```python
from build123d import *

# Parameters (mm, degrees)
SKETCH1_W                       = 88.9
SKETCH1_H                       = 60.325
BOSS_EXTRUDE1_DEPTH             = 36.5252
CUT_EXTRUDE1_DEPTH              = 30.1752
CUT_EXTRUDE5_DEPTH              = 4.7752
SKETCH3_R                       = 6.0452
CUT_EXTRUDE2_DEPTH              = 65.958980451
CUT_EXTRUDE3_DEPTH              = 3.6576
SKETCH8_OUTSIDE_W               = 113.594
SKETCH8_OUTSIDE_H               = 85.018
CUT_EXTRUDE4_DEPTH              = 28.575
F_10_32_TAPPED_HOLE1_AT_2_COUNT = 2
F_10_32_TAPPED_HOLE1_AT_2_PITCH = 47.6504
F_10_32_TAPPED_HOLE1_AT_3_COUNT = 2
F_10_32_TAPPED_HOLE1_AT_3_PITCH = 76.2
F_10_32_TAPPED_HOLE1_AT_4_COUNT = 2
F_10_32_TAPPED_HOLE1_AT_4_PITCH = 89.872134837
F_6_32_TAPPED_HOLE1_D           = 2.7051
F_6_32_TAPPED_HOLE1_DEPTH       = 9.398
F_6_32_TAPPED_HOLE1_CSINK_D     = 3.81
F_6_32_TAPPED_HOLE1_CSINK_ANGLE = 90
F_6_32_TAPPED_HOLE1_TIP         = 0.81269403
FILLET1_R                       = 3.175
F_8_32_TAPPED_HOLE1_AT_2_COUNT  = 2
F_8_32_TAPPED_HOLE1_AT_2_PITCH  = 9.525


with BuildPart() as part:
    # Sketch1 → Boss-Extrude1 (new body)
    with BuildSketch(Plane.XY):
        Rectangle(SKETCH1_W, SKETCH1_H)
    extrude(amount=-BOSS_EXTRUDE1_DEPTH)

    # Sketch2 → Cut-Extrude1 (cut)
    with BuildSketch(Plane.XY):
        with BuildLine():
            Line((8.699713209, 23.8252), (20.6375, 23.8252))
            ThreePointArc((20.6375, 23.8252), (32.202723567, 16.372637836), (30.194632556, 2.761515566))
            ThreePointArc((30.194632556, 2.761515566), (29.156922747, 0), (30.194632556, -2.761515566))
            ThreePointArc((30.194632556, -2.761515566), (32.202723567, -16.372637836), (20.6375, -23.8252))
            Line((20.6375, -23.8252), (8.699713209, -23.8252))
            Line((8.699713209, -23.8252), (-8.699713209, -23.8252))
            Line((-8.699713209, -23.8252), (-20.6375, -23.8252))
            ThreePointArc((-20.6375, -23.8252), (-32.202723567, -16.372637836), (-30.194632556, -2.761515566))
            ThreePointArc((-30.194632556, -2.761515566), (-29.156922747, 0), (-30.194632556, 2.761515566))
            ThreePointArc((-30.194632556, 2.761515566), (-32.202723567, 16.372637836), (-20.6375, 23.8252))
            Line((-20.6375, 23.8252), (-8.699713209, 23.8252))
            Line((-8.699713209, 23.8252), (8.699713209, 23.8252))
        make_face()
    extrude(amount=-CUT_EXTRUDE1_DEPTH, mode=Mode.SUBTRACT)

    # Sketch9 → Cut-Extrude5 (cut)
    with BuildSketch(Plane.XY):
        with BuildLine():
            Line((-20.6375, -25.4254), (20.6375, -25.4254))
            ThreePointArc((20.6375, -25.4254), (28.764361073, -22.891671397), (34.011365871, -16.188344448))
            Line((34.011365871, -16.188344448), (39.288861577, -2.248287943))
            ThreePointArc((39.288861577, -2.248287943), (39.7002, 0), (39.288861577, 2.248287943))
            Line((39.288861577, 2.248287943), (34.011365871, 16.188344448))
            ThreePointArc((34.011365871, 16.188344448), (28.764361073, 22.891671397), (20.6375, 25.4254))
            Line((20.6375, 25.4254), (-20.6375, 25.4254))
            ThreePointArc((-20.6375, 25.4254), (-28.764361073, 22.891671397), (-34.011365871, 16.188344448))
            Line((-34.011365871, 16.188344448), (-39.288861577, 2.248287943))
            ThreePointArc((-39.288861577, 2.248287943), (-39.7002, 0), (-39.288861577, -2.248287943))
            Line((-39.288861577, -2.248287943), (-34.011365871, -16.188344448))
            ThreePointArc((-34.011365871, -16.188344448), (-28.764361073, -22.891671397), (-20.6375, -25.4254))
        make_face()
    extrude(amount=-CUT_EXTRUDE5_DEPTH, mode=Mode.SUBTRACT)

    # Sketch3 → Cut-Extrude2 (cut, through all)
    with BuildSketch(Plane(origin=(0, 0, -36.5252), x_dir=(-1, 0, 0), z_dir=(0, 0, -1))):
        with Locations((-20.6502, 11.1252)):
            Circle(SKETCH3_R)
        with Locations((-20.6502, -11.1252)):
            Circle(SKETCH3_R)
        with Locations((20.6502, 11.1252)):
            Circle(SKETCH3_R)
        with Locations((20.6502, -11.1252)):
            Circle(SKETCH3_R)
    extrude(amount=-CUT_EXTRUDE2_DEPTH, mode=Mode.SUBTRACT)

    # Sketch4 → Cut-Extrude3 (cut)
    with BuildSketch(Plane.XY):
        with BuildLine():
            Line((20.6375, 28.9814), (-20.6375, 28.9814))
            ThreePointArc((-20.6375, 28.9814), (-30.78525015, 25.817614551), (-37.337016354, 17.447385697))
            Line((-37.337016354, 17.447385697), (-42.61451206, 3.507329192))
            ThreePointArc((-42.61451206, 3.507329192), (-43.2562, 0), (-42.61451206, -3.507329192))
            Line((-42.61451206, -3.507329192), (-37.337016354, -17.447385697))
            ThreePointArc((-37.337016354, -17.447385697), (-30.78525015, -25.817614551), (-20.6375, -28.9814))
            Line((-20.6375, -28.9814), (20.6375, -28.9814))
            ThreePointArc((20.6375, -28.9814), (30.78525015, -25.817614551), (37.337016354, -17.447385697))
            Line((37.337016354, -17.447385697), (42.61451206, -3.507329192))
            ThreePointArc((42.61451206, -3.507329192), (43.2562, 0), (42.61451206, 3.507329192))
            Line((42.61451206, 3.507329192), (37.337016354, 17.447385697))
            ThreePointArc((37.337016354, 17.447385697), (30.78525015, 25.817614551), (20.6375, 28.9814))
        make_face()
    extrude(amount=-CUT_EXTRUDE3_DEPTH, mode=Mode.SUBTRACT)

    # Sketch8 outside → Cut-Extrude4 (cut)
    with BuildSketch(Plane(origin=(0, 0, -36.5252), x_dir=(-1, 0, 0), z_dir=(0, 0, -1))):
        Rectangle(SKETCH8_OUTSIDE_W, SKETCH8_OUTSIDE_H)
        with BuildLine():
            Line((20.6375, -28.6512), (-20.6375, -28.6512))
            ThreePointArc((-20.6375, -28.6512), (-33.030253447, -23.517953447), (-38.1635, -11.1252))
            Line((-38.1635, -11.1252), (-38.1635, 11.1252))
            ThreePointArc((-38.1635, 11.1252), (-33.030253447, 23.517953447), (-20.6375, 28.6512))
            Line((-20.6375, 28.6512), (20.6375, 28.6512))
            ThreePointArc((20.6375, 28.6512), (33.030253447, 23.517953447), (38.1635, 11.1252))
            Line((38.1635, 11.1252), (38.1635, -11.1252))
            ThreePointArc((38.1635, -11.1252), (33.030253447, -23.517953447), (20.6375, -28.6512))
        make_face(mode=Mode.SUBTRACT)
    extrude(amount=-CUT_EXTRUDE4_DEPTH, mode=Mode.SUBTRACT)

    # Sketch6 → #10-32 Tapped Hole1 (revolve, cut)
    with BuildSketch(Plane(origin=(38.1, 23.8252, 0), x_dir=(0, -1, 0), z_dir=(1, 0, 0))):
        Polygon((0, 0), (0, 7.9502), (2.667, 7.9502), (2.0193, 7.3025), (2.0193, 0.6477), (2.667, 0), align=None)
    f_10_32_tapped_hole1 = revolve(axis=Axis((38.1, 23.8252, 6.35), (0, 0, -1)), mode=Mode.SUBTRACT)

    # #10-32 Tapped Hole1 at 2: #10-32 Tapped Hole1 ×2
    with Locations(*[(0, -i * F_10_32_TAPPED_HOLE1_AT_2_PITCH, 0) for i in range(1, F_10_32_TAPPED_HOLE1_AT_2_COUNT)]):
        add(f_10_32_tapped_hole1, mode=Mode.SUBTRACT)

    # #10-32 Tapped Hole1 at 3: #10-32 Tapped Hole1 ×2
    with Locations(*[(-i * F_10_32_TAPPED_HOLE1_AT_3_PITCH, 0, 0) for i in range(1, F_10_32_TAPPED_HOLE1_AT_3_COUNT)]):
        add(f_10_32_tapped_hole1, mode=Mode.SUBTRACT)

    # #10-32 Tapped Hole1 at 4: #10-32 Tapped Hole1 ×2
    with Locations(*[Vector(-0.8478712577397053, -0.5302021598398957, 0) * (i * F_10_32_TAPPED_HOLE1_AT_4_PITCH) for i in range(1, F_10_32_TAPPED_HOLE1_AT_4_COUNT)]):
        add(f_10_32_tapped_hole1, mode=Mode.SUBTRACT)

    # #6-32 Tapped Hole1
    with Locations(Plane.XY.offset(-4.7752)):
        with Locations((33.3502, 0), (-33.3502, 0)):
            CounterSinkHole(F_6_32_TAPPED_HOLE1_D / 2, F_6_32_TAPPED_HOLE1_CSINK_D / 2, depth=F_6_32_TAPPED_HOLE1_DEPTH, counter_sink_angle=F_6_32_TAPPED_HOLE1_CSINK_ANGLE)
            with Locations((0, 0, -(F_6_32_TAPPED_HOLE1_DEPTH + F_6_32_TAPPED_HOLE1_TIP / 2))):  # 118° drill point
                Cone(0, F_6_32_TAPPED_HOLE1_D / 2, F_6_32_TAPPED_HOLE1_TIP, mode=Mode.SUBTRACT)

    # Fillet1
    fillet1_edges = [part.edges().sort_by_distance(p)[0] for p in [
        (-44.45, -30.1625, -3.9751),
        (44.45, -30.1625, -3.9751),
        (44.45, 30.1625, -3.9751),
        (-44.45, 30.1625, -3.9751),
    ]]
    fillet(fillet1_edges, radius=FILLET1_R)

    # Sketch14 → #8-32 Tapped Hole1 (revolve, cut)
    with BuildSketch(Plane(origin=(-6.35, 15.875, -30.1752), x_dir=(0, -1, 0), z_dir=(1, 0, 0))):
        Polygon((0, 0), (0, 6.35), (2.286, 6.35), (1.7272, 5.7912), (1.7272, 0.5588), (2.286, 0), align=None)
    f_8_32_tapped_hole1 = revolve(axis=Axis((-6.35, 15.875, -23.8252), (0, 0, -1)), mode=Mode.SUBTRACT)

    # #8-32 Tapped Hole1 at 2: #8-32 Tapped Hole1 ×2
    with Locations(*[(i * F_8_32_TAPPED_HOLE1_AT_2_PITCH, 0, 0) for i in range(1, F_8_32_TAPPED_HOLE1_AT_2_COUNT)]):
        add(f_8_32_tapped_hole1, mode=Mode.SUBTRACT)


solid = part.part
```
The listing builds one solid part. Answer for the finished solid, in the listing's coordinates (mm). A direction names the side the tool comes from. Give positions to 0.01 mm unless a question says otherwise; leave off trailing zeros. Loops run counter-clockwise (first coordinate to the right, second up) from the corner with the lowest first, then second, coordinate; pieces in that order, holes last. Notation, with made-up numbers: M -22.5,69 L 14.5,69 A20 ccw 14.5,74 Z; hole C -8.5,64 d1. An arc over 180 degrees is marked long. One line per item, written item: value.
1. For faces 1 (the face through (38.164, 0, -22)), 2 (the face through (-1, 30.162, -4)), 3 (the face through (0, 23.825, -17)), determine the directions among +Z, -Z, +X, -X, +Y, -Y from which every point of the face is accessible in a straight line to the end or side of a thin tool.
Found:
face 1: -Z, +X, +Y, -Y
face 2: +Z, -Z, +X, -X, +Y
face 3: +Z
2. Section A-A on y = -9 is taken. Determine the outline of the cut face in (x, z).
Found:
outline: M -44.45,-7.95 L -38.16,-7.95 L -38.16,-36.53 L -26.31,-36.53 L -26.31,-30.18 L -33.16,-30.18 L -33.16,-4.78 L -36.73,-4.78 L -36.73,-3.66 L -40.54,-3.66 L -40.54,0 L -44.45,0 Z; M -14.99,-36.53 L 14.99,-36.53 L 14.99,-30.18 L -14.99,-30.18 Z; M 26.31,-36.53 L 38.16,-36.53 L 38.16,-7.95 L 44.45,-7.95 L 44.45,0 L 40.54,0 L 40.54,-3.66 L 36.73,-3.66 L 36.73,-4.78 L 33.16,-4.78 L 33.16,-30.18 L 26.31,-30.18 Z
3. Find the intervals of material crossed by probe 1 along Y at (x, z) = (14, -5.5); probe 2 along Y at (x, z) = (-11, -29); probe 3 along X at (y, z) = (-16.5, -31), in increasing order.
Found:
probe 1: -30.16 to -23.83, 23.83 to 30.16
probe 2: -28.65 to -23.83, 23.83 to 28.65
probe 3: -37.32 to -23.42, -17.88 to 17.88, 23.42 to 37.32
4. Section C-C on z = -32 is taken. State how many separate pieces and enclosed holes the cut face has, plus the area to 3 significant figures.
Found:
separate pieces: 1
enclosed holes: 6
area: 3,630 mm^2
5. Section D-D on z = -24.5 is taken. Determine the outline of the cut face in (x, y).
Found:
outline: M -38.16,-11.13 A17.53 ccw -20.64,-28.65 L 20.64,-28.65 A17.53 ccw 38.16,-11.13 L 38.16,11.13 A17.53 ccw 20.64,28.65 L -20.64,28.65 A17.53 ccw -38.16,11.13 Z; hole M -30.19,-2.76 A12.7 ccw -20.64,-23.83 L 20.64,-23.83 A12.7 ccw 30.19,-2.76 A4.19 cw 30.19,2.76 A12.7 ccw 20.64,23.83 L -20.64,23.83 A12.7 ccw -30.19,2.76 A4.19 cw Z
6. Each of these flat-tipped pins is pushed along its axis until it touches: P1, Ø24, axis at x = -8.5, y = -10.5, coming from the +Z side; P2, Ø8, axis at y = 2, z = -17, coming from the -X side; P3, Ø2, axis at y = 1, z = -16, coming from the +X side; P4, Ø3, axis at x = 3.175, y = 15.875, coming from the +Z side. Where does it stop, or does it pass through?
Found:
P1: z = -30.18
P2: x = -38.16
P3: x = 38.16
P4: through
7. Section B-B on x = -6.35 is taken. Determine the outline of the cut face in (y, z), plus the area to 3 significant figures.
Found:
outline: M -30.16,-7.95 L -28.65,-7.95 L -28.65,-36.53 L 13.59,-36.53 L 14.15,-35.97 L 14.15,-30.73 L 13.59,-30.18 L -23.83,-30.18 L -23.83,-4.78 L -25.43,-4.78 L -25.43,-3.66 L -28.98,-3.66 L -28.98,0 L -30.16,0 Z; M 17.6,-35.97 L 18.16,-36.53 L 28.65,-36.53 L 28.65,-7.95 L 30.16,-7.95 L 30.16,0 L 28.98,0 L 28.98,-3.66 L 25.43,-3.66 L 25.43,-4.78 L 23.83,-4.78 L 23.83,-30.18 L 18.16,-30.18 L 17.6,-30.73 Z
area: 615 mm^2
